```python
from build123d import *

# Parameters (mm, degrees)
SKETCH1_R = 0.79375


with BuildPart() as part:
    # Sweep1: sweep along a path in Sketch2
    with BuildLine(Plane(origin=(0, 0, 0), x_dir=(0, 0, -1), z_dir=(1, 0, 0))) as sweep1_path:
        Line((0, 0), (30.1625, 0))
        ThreePointArc((30.1625, 0), (34.016556239, 4.915970709), (28.322806453, 7.485354074))
        Line((28.322806453, 7.485354074), (18.911942386, 2.56210837))
        ThreePointArc((18.911942386, 2.56210837), (17.944168821, 2.398278597), (17.065046405, 2.834821429))
        ThreePointArc((17.065046405, 2.834821429), (14.2875, 3.96875), (11.509953595, 2.834821429))
        ThreePointArc((11.509953595, 2.834821429), (10.598111946, 2.393794506), (9.605185033, 2.593934671))
        Line((9.605185033, 2.593934671), (1.74625, 7.131292929))
    # Sketch1 → Sweep1 (sweep)
    with BuildSketch(Plane.XY):
        Circle(SKETCH1_R)
    sweep(path=sweep1_path.line)


solid = part.part
```
Read the model definition and answer for the solid it produces. Units are mm, in the model's axes. Coordinates: 2 decimals unless noted, no trailing zeros. Loops run counter-clockwise (first coordinate to the right, second up) from the corner with the lowest first, then second, coordinate; pieces in that order, holes last.
(1) The part is cut by section A-A (x = -0.2). Determine the outline of the cut face in (y, z).
Solution:
outline: (-0.77, -30.16) arc R4.74 ccw (long way) to (8.17, -27.97) - (3.24, -18.56) arc R0.82 cw to (3.38, -17.6) arc R4.74 ccw to (3.38, -10.97) arc R0.82 cw to (3.26, -9.99) - (7.8, -2.13) - (6.47, -1.36) - (1.93, -9.22) arc R2.36 ccw to (2.29, -12.05) arc R3.2 cw to (2.29, -16.53) arc R2.36 ccw to (1.88, -19.27) - (6.8, -28.68) arc R3.2 cw (long way) to (0.77, -30.16) - (0.77, 0) - (-0.77, 0) - close
(2) Consider line 1 along Z through (x, y) = (-0.05, 2); line 2 along Z through (x, y) = (0.5, 3.5); line 3 along Z through (x, y) = (-0.25, 5.25). Determine where each line is inside the solid, lowest interval first.
Solution:
line 1: z = -34.5 to -32.66, -19.55 to -16.84, -11.74 to -9.05
line 2: z = -34.72 to -33.48, -22.03 to -19.37, -17.25 to -11.33, -9.27 to -6.8
line 3: z = -34.71 to -33.11, -25.68 to -22.42, -6.51 to -3.5
(3) The mould has two halves that part along Z. Classify faces 1 (the face through (-0.1, 5.69, -23.19)), 2 (the face through (-0.01, 7.14, -1.75)), 3 (the face through (-0.172, 0.775, -15.292)): released by +Z, released by -Z, zero draft, split by the parting line, or undercut.
Solution:
face 1: undercut
face 2: released by +Z
face 3: zero draft
